Build history of the part. All positions in model axes, mm. A direction names the side the tool comes from. Round coordinates to 2 decimals unless told otherwise and drop trailing zeros. Order: outer loops, then holes, each group sorted by start corner. A loop starts at its lowest first (then second) coordinate and runs counter-clockwise, first axis right, second up. Notation, with made-up numbers: (86, 11) -> (114, 11) arc R16 cw to (114, 22) -> close; hole circle Ø6 at (28.5, 74). An arc over 180 degrees is marked (long way). Write item = value, one per line.
from build123d import *

# Parameters (mm, degrees)
SKETCH4_W           = 20
SKETCH4_H           = 70
BOSS_EXTRUDE2_DEPTH = 5
SKETCH5_W           = 7
SKETCH5_H           = 70
BOSS_EXTRUDE3_DEPTH = 10
SKETCH6_W           = 70
SKETCH6_H           = 1.998143523
CUT_EXTRUDE1_DEPTH  = 3
SKETCH8_W           = 10
SKETCH8_H           = 30
CUT_EXTRUDE2_DEPTH  = 74.484692283
FILLET3_START       = -1
FILLET3_DEPTH       = 6
FILLET3_2_DEPTH     = 5
FILLET4_R           = 5
SKETCH10_W          = 13.639904779
SKETCH10_H          = 5
CUT_EXTRUDE3_DEPTH  = 75.330343737
SKETCH11_W          = 70
SKETCH11_H          = 5
BOSS_EXTRUDE4_DEPTH = 20
SKETCH13_W          = 15
SKETCH13_H          = 30
CUT_EXTRUDE4_DEPTH  = 20
FILLET6_R           = 5


with BuildPart() as part:
    # Sketch4 → Boss-Extrude2 (new body)
    with BuildSketch(Plane(origin=(0, 0, 0), x_dir=(1, 0, 0), z_dir=(0, 1, 0))):
        with Locations((10, 35)):
            Rectangle(SKETCH4_W, SKETCH4_H)
    extrude(amount=BOSS_EXTRUDE2_DEPTH)

    # Sketch5 → Boss-Extrude3 (add)
    with BuildSketch(Plane(origin=(0, 5, 0), x_dir=(1, 0, 0), z_dir=(0, 1, 0))):
        with Locations((3.5, 35)):
            Rectangle(SKETCH5_W, SKETCH5_H)
    extrude(amount=BOSS_EXTRUDE3_DEPTH)

    # Sketch6 → Cut-Extrude1 (cut)
    with BuildSketch(Plane(origin=(7, 0, 0), x_dir=(0, 0, -1), z_dir=(1, 0, 0))):
        with Locations((35, 10.999071762)):
            Rectangle(SKETCH6_W, SKETCH6_H)
    extrude(amount=-CUT_EXTRUDE1_DEPTH, mode=Mode.SUBTRACT)

    # Sketch8 → Cut-Extrude2 (cut, through all)
    with BuildSketch(Plane(origin=(0, 5, 0), x_dir=(1, 0, 0), z_dir=(0, 1, 0))):
        with Locations((15, 35)):
            Rectangle(SKETCH8_W, SKETCH8_H)
    extrude(amount=-CUT_EXTRUDE2_DEPTH, mode=Mode.SUBTRACT)

    # Fillet3: read off the stored shape, not the designer's step
    # Fillet3 outline → Fillet3 (cut)
    with BuildSketch(Plane(origin=(0, 0, 0), x_dir=(1, 0, 0), z_dir=(0, 1, 0)).offset(FILLET3_START)):
        with BuildLine():
            Line((20, 50), (20, 55))
            ThreePointArc((20, 55), (18.535533906, 51.464466094), (15, 50))
            Line((15, 50), (20, 50))
        make_face()
        with BuildLine():
            Line((20, 20), (15, 20))
            ThreePointArc((15, 20), (18.535533906, 18.535533906), (20, 15))
            Line((20, 15), (20, 20))
        make_face()
    extrude(amount=FILLET3_DEPTH, mode=Mode.SUBTRACT)

    # Fillet3 2 outline → Fillet3 2 (add)
    with BuildSketch(Plane(origin=(0, 0, 0), x_dir=(1, 0, 0), z_dir=(0, 1, 0))):
        with BuildLine():
            ThreePointArc((15, 20), (11.464466094, 21.464466094), (10, 25))
            Line((10, 25), (10, 20))
            Line((10, 20), (15, 20))
        make_face()
        with BuildLine():
            ThreePointArc((10, 45), (11.464466094, 48.535533906), (15, 50))
            Line((15, 50), (10, 50))
            Line((10, 50), (10, 45))
        make_face()
    extrude(amount=FILLET3_2_DEPTH)

    # Fillet4
    fillet4_edges = [part.edges().sort_by_distance(p)[0] for p in [
        (20, 2.5, -70),
        (20, 2.5, 0),
    ]]
    fillet(fillet4_edges, radius=FILLET4_R)

    # Sketch10 → Cut-Extrude3 (cut, through all)
    with BuildSketch(Plane(origin=(0, 0, -70), x_dir=(-1, 0, 0), z_dir=(0, 0, -1))):
        with Locations((-13.81995239, 2.5)):
            Rectangle(SKETCH10_W, SKETCH10_H)
    extrude(amount=-CUT_EXTRUDE3_DEPTH, mode=Mode.SUBTRACT)

    # Sketch11 → Boss-Extrude4 (add)
    with BuildSketch(Plane.ZY):
        with Locations((-35, 2.5)):
            Rectangle(SKETCH11_W, SKETCH11_H)
    extrude(amount=BOSS_EXTRUDE4_DEPTH)

    # Sketch13 → Cut-Extrude4 (cut)
    with BuildSketch(Plane(origin=(0, 5, 0), x_dir=(1, 0, 0), z_dir=(0, 1, 0))):
        with Locations((-12.5, 35)):
            Rectangle(SKETCH13_W, SKETCH13_H)
    extrude(amount=-CUT_EXTRUDE4_DEPTH, mode=Mode.SUBTRACT)

    # Fillet6
    fillet6_edges = [part.edges().sort_by_distance(p)[0] for p in [
        (-20, 2.5, -50),
        (-20, 2.5, -20),
        (-5, 2.5, -20),
        (-5, 2.5, -50),
    ]]
    fillet(fillet6_edges, radius=FILLET6_R)


solid = part.part
Q1. Probe probe 1 along Z at (x, y) = (-9.75, 2); probe 2 along X at (y, z) = (4.5, -38); probe 3 along X at (y, z) = (14, -46). List the from-to ranges inside material, lowest first.
Check values:
probe_1 = -70 to -49.99, -20.01 to 0
probe_2 = -5 to 7
probe_3 = 0 to 7
Q2. Cut at C-C, the plane y = 1.25. List the corners of the cut face in (x, z).
Check values:
outline = (-20, -70) -> (7, -70) -> (7, 0) -> (-20, 0) -> (-20, -15) arc R5 ccw to (-15, -20) -> (-10, -20) arc R5 cw to (-5, -25) -> (-5, -45) arc R5 cw to (-10, -50) -> (-15, -50) arc R5 ccw to (-20, -55) -> close
Q3. Mould opens along Z. For faces 4 (the face through (-13, 3, -50)), 5 (the face through (-5, 3, -35)), 6 (the face through (4, 11, -35)), 7 (the face through (-3, 4, 0)) say: released by +Z, released by -Z, zero draft, split by the parting line, or undercut.
Check values:
face_4 = undercut
face_5 = undercut
face_6 = zero draft
face_7 = released by +Z
Q4. Cut at A-A, the plane x = -11.75. List the corners of the cut face in (y, z).
Check values:
outline = (0, -70) -> (5, -70) -> (5, -50) -> (0, -50) -> close; (0, -20) -> (5, -20) -> (5, 0) -> (0, 0) -> close
Q5. Cut at B-B, the plane z = -9. List the corners of the cut face in (x, y), and give its area (3 significant figures).
Check values:
outline = (-20, 0) -> (7, 0) -> (7, 10) -> (4, 10) -> (4, 12) -> (7, 12) -> (7, 15) -> (0, 15) -> (0, 5) -> (-20, 5) -> close
area = 199 mm²
Q6. Cut at D-D, the plane x = -8.75. List the corners of the cut face in (y, z), and give its area (3 significant figures).
Check values:
outline = (0, -70) -> (5, -70) -> (5, -49.84) -> (0, -49.84) -> close; (0, -20.16) -> (5, -20.16) -> (5, 0) -> (0, 0) -> close
area = 202 mm²
Q7. Flat gauge pins, fed straight in: pin 1 (1 mm diameter, centred on y = 1.5, z = -34.5, fed in from -X); pin 2 (10 mm diameter, centred on x = -8.5, z = -29, fed in from +Y); pin 3 (0.6 mm diameter, centred on y = 11, z = -27.5, fed in from +X). Where does each tip first touch, or does it go through?
Check values:
pin_1 = -5
pin_2 = 5
pin_3 = 4
Q8. Which spindle directions (+Z, -Z, +X, -X, +Y, -Y) get a long thin tool onto all of the face, cutting with end or side? Do faces 1 (the face through (0, 10, -35)), 2 (the face through (6, 10, -35)), 3 (the face through (-13, 3, -20)). Say none if no direction does.
Check values:
face_1 = +Z, -Z, -X, +Y
face_2 = +Z, -Z, +X
face_3 = -X, +Y, -Y
